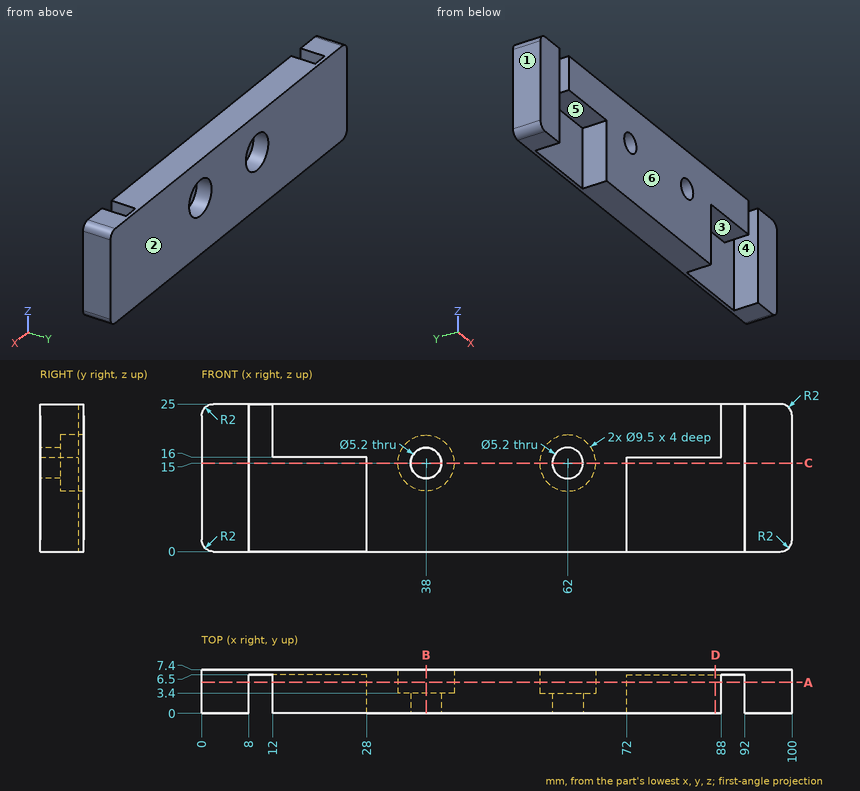
The drawing under review shows one solid part. Ordinate dimensions are in mm from its lowest x, y, z. A direction names the side the tool comes from. Give positions to 0.01 mm unless a question says otherwise; leave off trailing zeros. Loops run counter-clockwise (first coordinate to the right, second up) from the corner with the lowest first, then second, coordinate; pieces in that order, holes last. Notation, with made-up numbers: M 66,22.5 L 86,22.5 A21 ccw 86,50.5 Z; hole C -40,20.5 d1. An arc over 180 degrees is marked long. One line per item, written item: value. Start each with the question number.
Q1. Add section C-C (z = 15). Give the boundary of the cut face in (x, y).
Q2. Clearance check with flat-ended pins moving along their axes: pin 1 Ø10.5 at (x, z) = (37, 17) entering from +Y; pin 2 Ø6 at (x, z) = (38, 15) entering from +Y; pin 3 Ø5 at (x, z) = (21, 6) entering from -Y; pin 4 Ø3 at (x, y) = (80.5, 4) entering from -Z. State where each tip first meets the part, or that it passes through.
Q3. Machinability: for the marked faces 4, 5 and 6, which of the approach directions +Z, -Z, +X, -X, +Y, -Y give a long, thin tool a straight path to every point of the face, cutting with its end or side? Answer none if there is none.
Q4. Add section D-D (x = 87). Give the boundary of the cut face in (y, z), and give its area (3 significant figures).
Q5. Add section A-A (y = 5.25). Give the boundary of the cut face in (x, z), and give its area (3 significant figures).
Q6. Draft analysis for pull direction X (two halves, no side actions). For the marked faces 1, 2 and 3, state which applies: released by +X, released by -X, zero draft, split by the parting line, or undercut.
Q7. For L1, parallel to X at y = 3.5, z = 3.75; L2, parallel to X at y = 1.1, z = 15; L3, parallel to X at y = 5.85, z = 15, list the stretches that pass through material, from the lowest coordinate up.
Q8. Add section B-B (x = 38). Give the boundary of the cut face in (y, z).
Reply:
1. outline: M 0,0 L 8,0 L 8,6.5 L 28,6.5 L 28,0 L 35.4,0 L 35.4,3.4 L 33.25,3.4 L 33.25,7.4 L 0,7.4 Z; M 40.6,0 L 59.4,0 L 59.4,3.4 L 57.25,3.4 L 57.25,7.4 L 42.75,7.4 L 42.75,3.4 L 40.6,3.4 Z; M 64.6,0 L 72,0 L 72,6.5 L 92,6.5 L 92,0 L 100,0 L 100,7.4 L 66.75,7.4 L 66.75,3.4 L 64.6,3.4 Z
2. pin 1: y = 7.4
2. pin 2: y = 3.4
2. pin 3: y = 6.5
2. pin 4: z = 16
3. face 4: +Z, -Z, -Y
3. face 5: -Z, -Y
3. face 6: +Z, -Z, +X, -X, -Y
4. outline: M 0,16 L 6.5,16 L 6.5,0 L 7.4,0 L 7.4,25 L 0,25 Z
4. area: 81.0 mm²
5. outline: M 0,2 A2 ccw 2,0 L 8,0 L 8,25 L 2,25 A2 ccw 0,23 Z; M 12,16 L 28,16 L 28,0 L 72,0 L 72,16 L 88,16 L 88,25 L 12,25 Z; M 92,0 L 98,0 A2 ccw 100,2 L 100,23 A2 ccw 98,25 L 92,25 Z; hole C 38,15 d9.5; hole C 62,15 d9.5
5. area: 1,640 mm²
6. face 1: released by -X
6. face 2: zero draft
6. face 3: undercut
7. L1: 0 to 8, 28 to 72, 92 to 100
7. L2: 0 to 8, 28 to 35.4, 40.6 to 59.4, 64.6 to 72, 92 to 100
7. L3: 0 to 8, 28 to 33.25, 42.75 to 57.25, 66.75 to 72, 92 to 100
8. outline: M 0,0 L 7.4,0 L 7.4,10.25 L 3.4,10.25 L 3.4,12.4 L 0,12.4 Z; M 0,17.6 L 3.4,17.6 L 3.4,19.75 L 7.4,19.75 L 7.4,25 L 0,25 Z
